The model under review builds one solid part; all positions refer to its coordinate system, in mm. A direction names the side the tool comes from. Round coordinates to 2 decimals unless told otherwise and drop trailing zeros. Loops run counter-clockwise (first coordinate to the right, second up) from the corner with the lowest first, then second, coordinate; pieces in that order, holes last. Notation, with made-up numbers: M -23,-17.75 L 28,-17.75 A22 ccw 28,-8.75 Z; hole C 73,67.5 d8. An arc over 180 degrees is marked long. Answer as a JSON object with one key per item and string values. Group by question number.
Item 1: Consider section D-D (y = 11.5). Give the boundary of the cut face in (x, z), and give its area (3 significant figures).
Item 2: Consider section C-C (x = 34). Give the boundary of the cut face in (y, z), and give its area (3 significant figures).
Item 3: Insertion check: P1, Ø3, axis at y = 16.5, z = 1.5, coming from the +X side; P2, Ø1.9, axis at x = 32, z = 2.5, coming from the -Y side; P3, Ø1.9, axis at y = -20, z = 3.5, coming from the -X side. Each pin has a flat end and moves straight along its axis. Give the tip position at first contact, or say it passes through.
Item 4: Consider section B-B (x = -63.5). Give the boundary of the cut face in (y, z) (3 decimals), and give its area (3 significant figures).
Item 5: To check wall thickness, follow line 1 (X direction, y = -20, z = 4.5); line 2 (Y direction, x = 10, z = 2.75); line 3 (X direction, y = -21, z = 1). State the ranges of each line that lie inside material, in increasing order.
Item 6: Consider section A-A (y = 0). Give the boundary of the cut face in (x, z) (3 decimals).
Item 7: The part is to be moulded in two halves that separate along X. For faces 4 (the face through (50.8, 9, 3)), 5 (the face through (-50.8, 21, 3)), 6 (the face through (38.1, 21, 3)), 7 (the face through (-12, 0, 6.35)), say which applies: +X half, -X half, draft (parallel to the pull), parting line (faces both ways), or undercut.
Item 8: Tool access review of faces 1 (the face through (48, -14.288, 3)), 2 (the face through (12.7, 21, 3)), 3 (the face through (6, -17.462, 3)): name each direction out of +Z, -Z, +X, -X, +Y, -Y from which nothing blocks a thin tool from reaching the whole face with its end or side.
```python
from build123d import *

# Parameters (mm, degrees)
MASS_DEPTH          = 6.35
SKETCH4_R           = 3.175
CUT_EXTRUDE1_DEPTH  = 78.071449197
SKETCH3_W           = 12.7
SKETCH3_H           = 12.7
CUT_EXTRUDE2_DEPTH  = 78.071449197
LPATTERN1_COUNT     = 4
LPATTERN1_PITCH     = 25.4
SKETCH5_W           = 12.7
SKETCH5_H           = 9.525
CUT_EXTRUDE3_DEPTH  = 78.071449197
LPATTERN2_COUNT     = 2
LPATTERN2_PITCH     = 19.05
LPATTERN2_COL_COUNT = 2
LPATTERN2_COL_PITCH = 19.05


with BuildPart() as part:
    # Sketch1 → Mass (new body)
    with BuildSketch(Plane.XY):
        with BuildLine():
            Line((-50.8, -23.8125), (50.8, -23.8125))
            Line((50.8, -23.8125), (50.8, 23.8125))
            Line((50.8, 23.8125), (-50.8, 23.8125))
            Line((-50.8, 23.8125), (-69.781543236, 7.160156393))
            ThreePointArc((-69.781543236, 7.160156393), (-73.025, 0), (-69.781543236, -7.160156393))
            Line((-69.781543236, -7.160156393), (-50.8, -23.8125))
        make_face()
    extrude(amount=MASS_DEPTH)

    # Sketch4 → Cut-Extrude1 (cut, through all)
    with BuildSketch(Plane(origin=(0, 0, 0), x_dir=(-1, 0, 0), z_dir=(0, 0, -1))):
        with Locations((63.5, 0)):
            Circle(SKETCH4_R)
    extrude(amount=-CUT_EXTRUDE1_DEPTH, mode=Mode.SUBTRACT)

    # Sketch3 → Cut-Extrude2 (cut, through all)
    with BuildSketch(Plane(origin=(0, 0, 0), x_dir=(-1, 0, 0), z_dir=(0, 0, -1))):
        with Locations((-31.75, 23.8125)):
            Rectangle(SKETCH3_W, SKETCH3_H)
        with Locations((-31.75, -23.8125)):
            Rectangle(SKETCH3_W, SKETCH3_H)
    cut_extrude2 = extrude(amount=-CUT_EXTRUDE2_DEPTH, mode=Mode.SUBTRACT)

    # LPattern1: Cut-Extrude2 ×4
    with Locations(*[(-i * LPATTERN1_PITCH, 0, 0) for i in range(1, LPATTERN1_COUNT)]):
        add(cut_extrude2, mode=Mode.SUBTRACT)

    # Sketch5 → Cut-Extrude3 (cut, through all)
    with BuildSketch(Plane(origin=(0, 0, 0), x_dir=(-1, 0, 0), z_dir=(0, 0, -1))):
        with Locations((-50.8, 0)):
            Rectangle(SKETCH5_W, SKETCH5_H)
    cut_extrude3 = extrude(amount=-CUT_EXTRUDE3_DEPTH, mode=Mode.SUBTRACT)

    # LPattern2: Cut-Extrude3 ×2
    with Locations(*[(0, -i * LPATTERN2_PITCH, 0) for i in range(1, LPATTERN2_COUNT)]):
        add(cut_extrude3, mode=Mode.SUBTRACT)

    # LPattern2 col: Cut-Extrude3 ×2
    with Locations(*[(0, i * LPATTERN2_COL_PITCH, 0) for i in range(1, LPATTERN2_COL_COUNT)]):
        add(cut_extrude3, mode=Mode.SUBTRACT)


solid = part.part
```
Geometry results:
{
 "1": {"outline": "M -64.83,0 L 50.8,0 L 50.8,6.35 L -64.83,6.35 Z", "area": "734 mm^2"},
 "2": {"outline": "M -17.46,0 L 17.46,0 L 17.46,6.35 L -17.46,6.35 Z", "area": "222 mm^2"},
 "3": {"P1": "stops at x = 44.45", "P2": "stops at y = -17.46", "P3": "stops at x = -56.23"},
 "4": {"outline": "M -12.671,0 L -3.175,0 L -3.175,6.35 L -12.671,6.35 Z; M 3.175,0 L 12.671,0 L 12.671,6.35 L 3.175,6.35 Z", "area": "121 mm^2"},
 "5": {"line 1": "x = -55.15 to -50.8, -38.1 to -25.4, -12.7 to 0, 12.7 to 25.4, 38.1 to 44.45", "line 2": "y = -17.46 to 17.46", "line 3": "x = -54.01 to -50.8, -38.1 to -25.4, -12.7 to 0, 12.7 to 25.4, 38.1 to 44.45"},
 "6": {"outline": "M -73.025,0 L -66.675,0 L -66.675,6.35 L -73.025,6.35 Z; M -60.325,0 L 44.45,0 L 44.45,6.35 L -60.325,6.35 Z"},
 "7": {"face 4": "+X half", "face 5": "undercut", "face 6": "undercut", "face 7": "draft"},
 "8": {"face 1": "+Z, -Z, +X, -Y", "face 2": "+Z, -Z, +Y", "face 3": "+Z, -Z, -Y"}
}
